```python
from build123d import *

# Parameters (mm, degrees)
SKETCH1_W                       = 55.88
SKETCH1_H                       = 25.4
EXTRUDE1_DEPTH                  = 101.6
SKETCH4_R                       = 9.525
CUT_EXTRUDE2_DEPTH              = 58.42
SKETCH7_W                       = 25.4
SKETCH7_H                       = 101.6
CUT_EXTRUDE5_DEPTH              = 12.7
SKETCH8_W                       = 25.4
SKETCH8_H                       = 101.6
CUT_EXTRUDE6_DEPTH              = 12.7
SKETCH15_W                      = 5.800046345
SKETCH15_H                      = 2.54
CUT_EXTRUDE10_DEPTH             = 58.42
F_27_0_144_DIAMETER_HOLE1_D     = 3.6576
F_27_0_144_DIAMETER_HOLE1_DEPTH = 13.97
F_27_0_144_DIAMETER_HOLE2_D     = 3.6576
F_27_0_144_DIAMETER_HOLE2_DEPTH = 13.97
F_6_32_TAPPED_HOLE1_D           = 2.7051
F_6_32_TAPPED_HOLE1_DEPTH       = 11.43
F_6_32_TAPPED_HOLE1_TIP         = 0.81269403
F_6_32_TAPPED_HOLE2_D           = 2.7051
F_6_32_TAPPED_HOLE2_DEPTH       = 11.43
F_6_32_TAPPED_HOLE2_TIP         = 0.81269403
SKETCH37_W                      = 25.4
SKETCH37_H                      = 38.1
CUT_EXTRUDE11_DEPTH             = 114.279443855
F_8_32_TAPPED_HOLE3_D           = 3.4544
CIRPATTERN2_COUNT               = 2
SKETCH44_W                      = 30.48
SKETCH44_H                      = 20.32
CUT_EXTRUDE12_DEPTH             = 107.02028155
CIRPATTERN3_COUNT               = 2
F_6_32_TAPPED_HOLE3_D           = 2.7051
F_6_32_TAPPED_HOLE3_DEPTH       = 13.97
F_6_32_TAPPED_HOLE4_D           = 2.7051
F_6_32_TAPPED_HOLE4_DEPTH       = 13.97
F_27_0_144_DIAMETER_HOLE3_D     = 3.6576
F_27_0_144_DIAMETER_HOLE3_DEPTH = 13.97
F_27_0_144_DIAMETER_HOLE4_D     = 3.6576
F_27_0_144_DIAMETER_HOLE4_DEPTH = 13.97


with BuildPart() as part:
    # Sketch1 → Extrude1 (new body)
    with BuildSketch(Plane(origin=(0, 0, 0), x_dir=(1, 0, 0), z_dir=(0, 1, 0))):
        with Locations((-1.27, -12.7)):
            Rectangle(SKETCH1_W, SKETCH1_H)
    extrude(amount=EXTRUDE1_DEPTH)

    # Sketch4 → Cut-Extrude2 (cut)
    with BuildSketch(Plane(origin=(0, 101.6, 0), x_dir=(-1, 0, 0), z_dir=(0, 1, 0))):
        with Locations(Location((1.27, 12.7, 0), (0, 0, 90))):
            Circle(SKETCH4_R)
    extrude(amount=-CUT_EXTRUDE2_DEPTH, mode=Mode.SUBTRACT)

    # Sketch7 → Cut-Extrude5 (cut)
    with BuildSketch(Plane(origin=(26.67, 0, 0), x_dir=(0, 0, -1), z_dir=(1, 0, 0))):
        with Locations((-12.7, 50.8)):
            Rectangle(SKETCH7_W, SKETCH7_H)
    extrude(amount=-CUT_EXTRUDE5_DEPTH, mode=Mode.SUBTRACT)

    # Sketch8 → Cut-Extrude6 (cut)
    with BuildSketch(Plane.ZY.offset(29.21)):
        with Locations((12.7, 50.8)):
            Rectangle(SKETCH8_W, SKETCH8_H)
    extrude(amount=-CUT_EXTRUDE6_DEPTH, mode=Mode.SUBTRACT)

    # Sketch15 → Cut-Extrude10 (cut)
    with BuildSketch(Plane(origin=(0, 101.6, 0), x_dir=(-1, 0, 0), z_dir=(0, 1, 0))):
        with Locations((-11.069976827, 12.7)):
            Rectangle(SKETCH15_W, SKETCH15_H)
    cut_extrude10 = extrude(amount=-CUT_EXTRUDE10_DEPTH, mode=Mode.SUBTRACT)

    # #27 (0.144) Diameter Hole1
    with Locations(Plane(origin=(11.43, 68.58, 0), x_dir=(-1, 0, 0), z_dir=(0, 0, -1))):
        with Locations((0, 0)):
            Hole(F_27_0_144_DIAMETER_HOLE1_D / 2, depth=F_27_0_144_DIAMETER_HOLE1_DEPTH)

    # #27 (0.144) Diameter Hole2
    with Locations(Plane(origin=(11.434321399, 55.88, 0), x_dir=(-1, 0, 0), z_dir=(0, 0, -1))):
        with Locations((0, 0)):
            Hole(F_27_0_144_DIAMETER_HOLE2_D / 2, depth=F_27_0_144_DIAMETER_HOLE2_DEPTH)

    # #6-32 Tapped Hole1
    with Locations(Plane(origin=(11.43, 68.58, 25.4), x_dir=(1, 0, 0), z_dir=(0, 0, 1))):
        with Locations((0, 0)):
            Hole(F_6_32_TAPPED_HOLE1_D / 2, depth=F_6_32_TAPPED_HOLE1_DEPTH)
            with Locations((0, 0, -(F_6_32_TAPPED_HOLE1_DEPTH + F_6_32_TAPPED_HOLE1_TIP / 2))):  # 118° drill point
                Cone(0, F_6_32_TAPPED_HOLE1_D / 2, F_6_32_TAPPED_HOLE1_TIP, mode=Mode.SUBTRACT)

    # #6-32 Tapped Hole2
    with Locations(Plane(origin=(11.43, 55.88, 25.4), x_dir=(1, 0, 0), z_dir=(0, 0, 1))):
        with Locations((0, 0)):
            Hole(F_6_32_TAPPED_HOLE2_D / 2, depth=F_6_32_TAPPED_HOLE2_DEPTH)
            with Locations((0, 0, -(F_6_32_TAPPED_HOLE2_DEPTH + F_6_32_TAPPED_HOLE2_TIP / 2))):  # 118° drill point
                Cone(0, F_6_32_TAPPED_HOLE2_D / 2, F_6_32_TAPPED_HOLE2_TIP, mode=Mode.SUBTRACT)

    # Sketch37 → Cut-Extrude11 (cut, through all)
    with BuildSketch(Plane.ZY.offset(29.21)):
        with Locations((12.7, 19.05)):
            Rectangle(SKETCH37_W, SKETCH37_H)
    extrude(amount=-CUT_EXTRUDE11_DEPTH, mode=Mode.SUBTRACT)

    # #8-32 Tapped Hole3 (through all)
    with Locations(Plane(origin=(-1.27, 38.1, 19.05), x_dir=(0, 0, -1), z_dir=(0, -1, 0))):
        with Locations((0, 0)):
            f_8_32_tapped_hole3 = Hole(F_8_32_TAPPED_HOLE3_D / 2)

    # CirPattern2: #8-32 Tapped Hole3 ×2 about axis
    cirpattern2_axis = Axis((-1.27, 0, 12.7), (0, 1, 0))
    for i in range(1, CIRPATTERN2_COUNT):
        add(f_8_32_tapped_hole3.rotate(cirpattern2_axis, i * 360 / CIRPATTERN2_COUNT), mode=Mode.SUBTRACT)

    # Sketch44 → Cut-Extrude12 (cut, through all)
    with BuildSketch(Plane(origin=(0, 0, 0), x_dir=(-1, 0, 0), z_dir=(0, 0, -1))):
        with Locations((1.27, 91.44)):
            Rectangle(SKETCH44_W, SKETCH44_H)
    extrude(amount=-CUT_EXTRUDE12_DEPTH, mode=Mode.SUBTRACT)

    # CirPattern3: Cut-Extrude10 ×2 about axis
    cirpattern3_axis = Axis((-1.27, 87.197587188, 12.7), (0, 1, 0))
    for i in range(1, CIRPATTERN3_COUNT):
        add(cut_extrude10.rotate(cirpattern3_axis, i * 360 / CIRPATTERN3_COUNT), mode=Mode.SUBTRACT)

    # #6-32 Tapped Hole3
    with Locations(Plane(origin=(-13.97, 68.58, 25.4), x_dir=(1, 0, 0), z_dir=(0, 0, 1))):
        with Locations((0, 0)):
            Hole(F_6_32_TAPPED_HOLE3_D / 2, depth=F_6_32_TAPPED_HOLE3_DEPTH)

    # #6-32 Tapped Hole4
    with Locations(Plane(origin=(-13.97, 55.88, 25.4), x_dir=(1, 0, 0), z_dir=(0, 0, 1))):
        with Locations((0, 0)):
            Hole(F_6_32_TAPPED_HOLE4_D / 2, depth=F_6_32_TAPPED_HOLE4_DEPTH)

    # #27 (0.144) Diameter Hole3
    with Locations(Plane(origin=(-13.97, 68.58, 0), x_dir=(-1, 0, 0), z_dir=(0, 0, -1))):
        with Locations((0, 0)):
            Hole(F_27_0_144_DIAMETER_HOLE3_D / 2, depth=F_27_0_144_DIAMETER_HOLE3_DEPTH)

    # #27 (0.144) Diameter Hole4
    with Locations(Plane(origin=(-13.97, 55.88, 0), x_dir=(-1, 0, 0), z_dir=(0, 0, -1))):
        with Locations((0, 0)):
            Hole(F_27_0_144_DIAMETER_HOLE4_D / 2, depth=F_27_0_144_DIAMETER_HOLE4_DEPTH)


solid = part.part
```
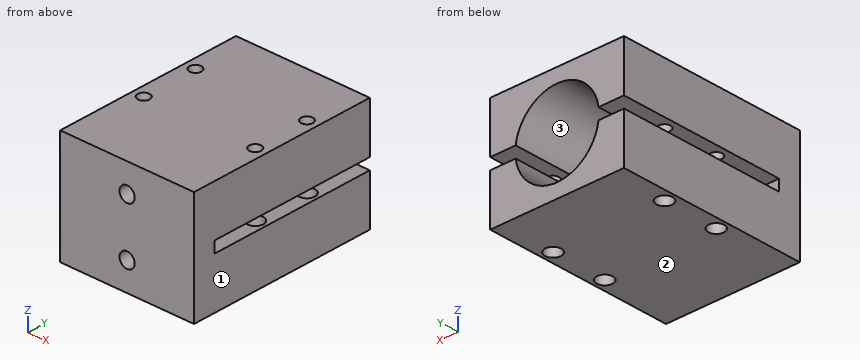
Here's how the part is built. I have some questions about the finished solid (model axes, mm). Face numbers are marked on the shaded views. Give positions to 0.01 mm unless a question says otherwise; leave off trailing zeros. Order: outer loops, then holes, each group sorted by start corner. A loop starts at its lowest first (then second) coordinate and runs counter-clockwise, first axis right, second up. Notation, with made-up numbers: M 1,48.25 L 44,48.25 A5 ccw 44,55.25 Z; hole C 25,-19 d7. An arc over 180 degrees is marked long. Use a Markdown table: item, result. Add a question column.
1. For pin 1 Ø4.5 at (x, y) = (12, 63) entering from -Z; pin 2 Ø3.5 at (x, y) = (11.43, 68.58) entering from -Z; pin 3 Ø3 at (x, z) = (-1.27, 19.05) entering from -Y; pin 4 Ø5.5 at (x, z) = (-2, 17) entering from +Y, each with a flat end and sliding along its axis, tell me the tip position at first contact or that it passes through.
2. Suppose I cut it at D-D (x = -13.97). List the corners of the cut face in (y, z) for me, and give its area (3 significant figures).
3. Suppose I cut it at A-A (z = 6.35). List the corners of the cut face in (x, y) for me, and give its area (3 significant figures).
4. Suppose I cut it at B-B (y = 68.58). List the corners of the cut face in (x, z) for me (3 decimals), and give its area (3 significant figures).
5. If we mould it in two halves opening along Z, with no side actions, what happens to the marked faces 1, 2 and 3? For each: +Z half, -Z half, draft (parallel to the pull), parting line (faces both ways), or undercut.
6. Suppose I cut it at C-C (z = 23.5). List the corners of the cut face in (x, y) for me.
7. I need wall thicknesses on probe 1 along Y at (x, z) = (-14, 19.5); probe 2 along X at (y, z) = (68.58, 2.5); probe 3 along Y at (x, z) = (11, 16.5). Which ranges of each line are inside material? Lowest first, please. Write a range as from..to.
Results list:
| question | item | result |
|---|---|---|
| 1 | pin 1 | stops at z = 0 |
| 1 | pin 2 | stops at z = 13.97 |
| 1 | pin 3 | passes through |
| 1 | pin 4 | stops at y = 43.18 |
| 2 | outline | M 38.1,0 L 54.05,0 L 54.05,11.43 L 43.18,11.43 L 43.18,13.97 L 54.53,13.97 L 54.53,25.4 L 38.1,25.4 Z; M 57.23,13.97 L 67.23,13.97 L 67.23,25.4 L 57.23,25.4 Z; M 57.71,0 L 66.75,0 L 66.75,11.43 L 57.71,11.43 Z; M 69.93,13.97 L 81.28,13.97 L 81.28,25.4 L 69.93,25.4 Z; M 70.41,0 L 81.28,0 L 81.28,11.43 L 70.41,11.43 Z |
| 2 | area | 855 mm² |
| 3 | outline | M -16.51,38.1 L -3,38.1 L -3,43.18 L -8.37,43.18 L -8.37,81.28 L -16.51,81.28 Z; M 0.46,38.1 L 13.97,38.1 L 13.97,81.28 L 5.83,81.28 L 5.83,43.18 L 0.46,43.18 Z; hole C -13.97,55.88 d3.66; hole C -13.97,68.58 d3.66; hole C 11.43,68.58 d3.66; hole C 11.43,55.88 d3.66 |
| 3 | area | 716 mm² |
| 4 | outline | M -16.51,0 L -15.799,0 L -15.799,11.43 L -16.51,11.43 Z; M -16.51,13.97 L -15.323,13.97 L -15.323,25.4 L -16.51,25.4 Z; M -12.617,13.97 L -10.71,13.97 A9.525 cw 8.17,13.97 L 10.077,13.97 L 10.077,25.4 L -12.617,25.4 Z; M -12.141,0 L 9.601,0 L 9.601,11.43 L 8.17,11.43 A9.525 cw -10.71,11.43 L -12.141,11.43 Z; M 12.783,13.97 L 13.97,13.97 L 13.97,25.4 L 12.783,25.4 Z; M 13.259,0 L 13.97,0 L 13.97,11.43 L 13.259,11.43 Z |
| 4 | area | 315 mm² |
| 5 | face 1 | draft |
| 5 | face 2 | -Z half |
| 5 | face 3 | undercut |
| 6 | outline | M -16.51,38.1 L 13.97,38.1 L 13.97,81.28 L -16.51,81.28 Z; hole C -13.97,55.88 d2.71; hole C -13.97,68.58 d2.71; hole C 11.43,55.88 d2.71; hole C 11.43,68.58 d2.71 |
| 7 | probe 1 | y = 38.1..54.53, 57.23..67.23, 69.93..81.28 |
| 7 | probe 2 | x = -16.51..-15.8, -12.14..9.6, 13.26..13.97 |
| 7 | probe 3 | y = 38.1..54.6, 57.16..67.3, 69.86..81.28 |
